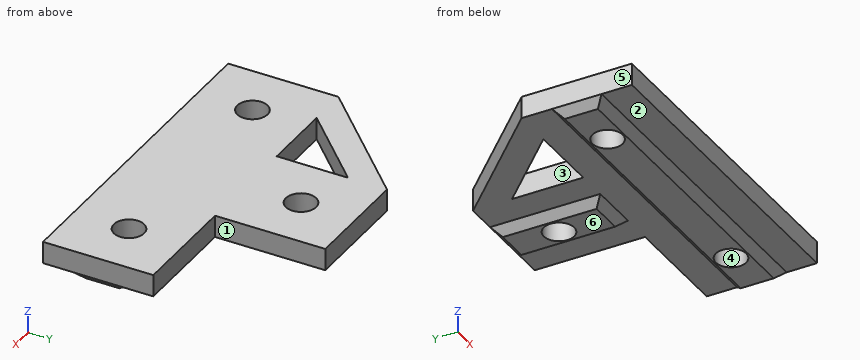
```python
from build123d import *

# Parameters (mm, degrees)
F1_DEPTH = 4
F3_DEPTH = 60
F5_DEPTH = 20
F6_SIZE  = 1.49999
F7_R     = 2.75
F8_DEPTH = 5.501


# Not quite as in the source:
# - a fillet or chamfer is up to 0.001 mm smaller than in the source, because OpenCascade refuses the exact size


with BuildPart() as f1:
    # F0 (on Top) → F1 (new body)
    with BuildSketch(Plane.XY):
        Polygon((0, 20), (0, 0), (60, 0), (60, 20), (40, 20), (40, 40), (20, 40), align=None)
        Polygon((20, 32.9289321881), (20, 20), (7.0710678119, 20), align=None, mode=Mode.SUBTRACT)
    extrude(amount=F1_DEPTH)

    # F2 (on face) → F3 (join, through all)
    with BuildSketch(Plane.YZ.offset(60)):
        Polygon((14.5, 0), (5.5, 0), (7, -1.5), (13, -1.5), align=None)
    extrude(amount=-F3_DEPTH)

    # F4 (on face) → F5 (join, through all)
    with BuildSketch(Plane(origin=(0, 40, 0), x_dir=(-1, 0, 0), z_dir=(0, 1, 0))):
        Polygon((-25.5, 0), (-34.5, 0), (-33, -1.5), (-27, -1.5), align=None)
    extrude(amount=-F5_DEPTH)

    # F6 (size 1.5 in the source; OpenCascade refuses exactly that, so slightly less here)
    f6_edges = [f1.edges().sort_by_distance(p)[0] for p in [
        (60, 10, -1.5),
        (0, 10, -1.5),
        (30, 20, -1.5),
        (30, 40, -1.5),
    ]]
    chamfer(f6_edges, length=F6_SIZE)

    # F7 (on face) → F8 (cut, through all)
    with BuildSketch(Plane.XY.offset(4)):
        with Locations((30, 30)):
            Circle(F7_R)
        with Locations((10, 10)):
            Circle(F7_R)
        with Locations((50, 10)):
            Circle(F7_R)
    extrude(amount=-F8_DEPTH, mode=Mode.SUBTRACT)


solid = f1.part
```
For this review, take the finished solid that the model builds, in its own axes (mm). Face numbers are marked on the shaded views. A direction names the side the tool comes from. Give positions to 0.01 mm unless a question says otherwise; leave off trailing zeros. Order: outer loops, then holes, each group sorted by start corner. A loop starts at its lowest first (then second) coordinate and runs counter-clockwise, first axis right, second up.
1) Take a section at A-A (y = 10). Give the boundary of the cut face in (x, z).
2) Wall thickness on line 1 (Y direction, x = 10, z = 0.7); line 2 (Y direction, x = 50, z = 2.75); line 3 (Z direction, x = 28.5, y = 4.5): over which ranges is each line inside the solid? List them lowest first.
3) For the marked faces 1, 2 and 3, list the 3-axis set-ups (+Z, -Z, +X, -X, +Y, -Y) from which the entire face can be reached by the end or side of a thin tool; tool diameter is ignored.
4) Take a section at B-B (z = -0.8). Give the boundary of the cut face in (x, y).
5) The part is to be moulded in two halves that separate along X. For the marked faces 4, 5 and 6, say which applies: released by +X, released by -X, zero draft, split by the parting line, or undercut.
6) Take a section at C-C (x = 50). Give the boundary of the cut face in (y, z), then the cut area to 3 significant figures.
7) Take a section at D-D (z = 3.05). Give the boundary of the cut face in (x, y), then the cut area to 3 significant figures.
8) Insertion check: pin 1 (4 mm diameter, centred on x = 41, y = 19.5, fed in from -Z); pin 2 (2 mm diameter, centred on y = 25, z = 1.5, fed in from +X); pin 3 (2 mm diameter, centred on x = 54, z = 1, fed in from +Y). Each pin has a flat end and moves straight along its axis. Give the tip position at first contact, or say it passes through.
Derived:
1. outline: (0, 0) - (1.5, -1.5) - (7.25, -1.5) - (7.25, 4) - (0, 4) - close; (12.75, -1.5) - (47.25, -1.5) - (47.25, 4) - (12.75, 4) - close; (52.75, -1.5) - (58.5, -1.5) - (60, 0) - (60, 4) - (52.75, 4) - close
2. line 1: y = 0 to 7.25, 12.75 to 20, 22.93 to 30
2. line 2: y = 0 to 7.25, 12.75 to 20
2. line 3: z = 0 to 4
3. face 1: +Z, -Z, +X, +Y
3. face 2: -Z, +X, -X, -Y
3. face 3: +Z, -Z
4. outline: (0.8, 6.3) - (59.2, 6.3) - (59.2, 13.7) - (0.8, 13.7) - close; (26.3, 20.8) - (33.7, 20.8) - (33.7, 39.2) - (26.3, 39.2) - close; hole circle Ø5.5 at (10, 10); hole circle Ø5.5 at (30, 30); hole circle Ø5.5 at (50, 10)
5. face 4: undercut
5. face 5: released by -X
5. face 6: zero draft
6. outline: (0, 0) - (5.5, 0) - (7, -1.5) - (7.25, -1.5) - (7.25, 4) - (0, 4) - close; (12.75, -1.5) - (13, -1.5) - (14.5, 0) - (20, 0) - (20, 4) - (12.75, 4) - close
6. area: 61.0 mm2
7. outline: (0, 0) - (60, 0) - (60, 20) - (40, 20) - (40, 40) - (20, 40) - (0, 20) - close; hole (7.07, 20) - (20, 20) - (20, 32.93) - close; hole circle Ø5.5 at (10, 10); hole circle Ø5.5 at (30, 30); hole circle Ø5.5 at (50, 10)
7. area: 1,650 mm2
8. pin 1: stops at z = 0
8. pin 2: stops at x = 40
8. pin 3: stops at y = 20
